Build history of the part. All positions in model axes, mm. Give positions to 0.01 mm unless a question says otherwise; leave off trailing zeros. Write each loop counter-clockwise with the first axis right and the second up, starting at its lowest first coordinate (ties: lowest second). Pieces come first, ordered by that corner, then holes. Notation, with made-up numbers: (-1.5, 30) -> (25.5, 30) arc R12 ccw to (25.5, 46) -> close; hole circle Ø6 at (-5, -16.75). An arc over 180 degrees is marked (long way). Put each result on its own line as item: value.
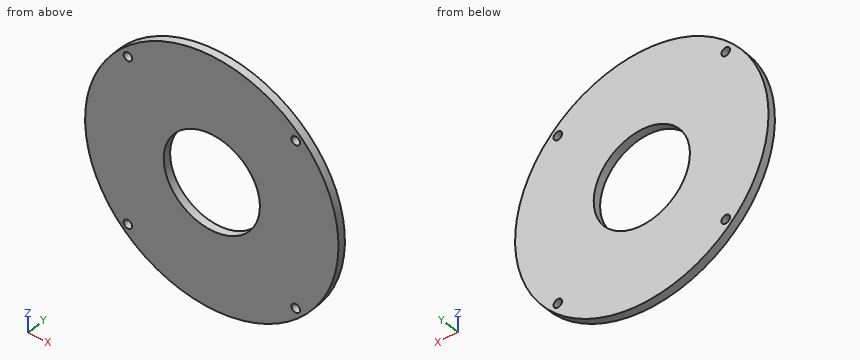
from build123d import *

# Parameters (mm, degrees)
SKETCH1_R            = 50.165
SKETCH1_R_2          = 19.05
BOSS_EXTRUDE1_DEPTH  = 1.5875
M3_CLEARANCE_HOLE1_D = 3.4


with BuildPart() as part:
    # Sketch1 → Boss-Extrude1 (new, symmetric)
    with BuildSketch(Plane(origin=(0, 0, 0), x_dir=(1, 0, 0), z_dir=(0, 1, 0))):
        with Locations(Location((0, 0, 0), (0, 0, 270))):
            Circle(SKETCH1_R)
        with Locations(Location((0, 0, 0), (0, 0, 270))):
            Circle(SKETCH1_R_2, mode=Mode.SUBTRACT)
    extrude(amount=BOSS_EXTRUDE1_DEPTH, both=True)

    # M3 Clearance Hole1 (through all)
    with Locations(Plane(origin=(0, 1.5875, 0), x_dir=(1, 0, 0), z_dir=(0, 1, 0))):
        with Locations((-33.226947648, -33.226947648), (-33.226947648, 33.226947648), (33.226947648, 33.226947648), (33.226947648, -33.226947648)):
            Hole(M3_CLEARANCE_HOLE1_D / 2)


solid = part.part
1) Slice it at D-D (z = 44). Write the cut outline in (x, y).
Filled sheet:
outline: (-24.09, -1.59) -> (24.09, -1.59) -> (24.09, 1.59) -> (-24.09, 1.59) -> close
2) Slice it at C-C (y = -0.8). Write the cut outline in (x, z) (3 decimals).
Filled sheet:
outline: circle Ø100.33 at (0, 0); hole circle Ø3.4 at (-33.227, -33.227); hole circle Ø3.4 at (-33.227, 33.227); hole circle Ø38.1 at (0, 0); hole circle Ø3.4 at (33.227, -33.227); hole circle Ø3.4 at (33.227, 33.227)
3) Pin check, flat tip, straight feed: pin 1 (1.5 mm diameter, centred on y = 0, z = 13, fed in from -X). Stop position of the tip, or through.
Filled sheet:
pin 1: x = -48.65
4) Wall check: L1, parallel to X at y = -1.35, z = -34.5; L2, parallel to X at y = 0.9, z = -33; L3, parallel to X at y = 1.2, z = -5. Give the ranges that are in metal, low to high.
Filled sheet:
L1: -36.42 to -34.35, -32.1 to 32.1, 34.35 to 36.42
L2: -37.78 to -34.91, -31.54 to 31.54, 34.91 to 37.78
L3: -49.92 to -18.38, 18.38 to 49.92
